```python
from build123d import *

# Parameters (mm, degrees)
F0_R         = 11.125
F1_DEPTH     = 10
F2_T1_DEPTH  = 17.5952575274
F2_T3_DEPTH  = 17.5952575274
F2_T6_ANGLE  = 359.64
F2_T8_ANGLE  = 359.64
F2_T10_ANGLE = 158.7108465942
F2_T12_ANGLE = 359.64
F2_T14_ANGLE = 359.64
F2_T16_ANGLE = 359.64
F2_T18_ANGLE = 359.64
F2_T20_ANGLE = 158.7108465942
F2_T22_ANGLE = 359.64
F2_T24_ANGLE = 359.64
F2_T26_ANGLE = 359.64
F2_T28_ANGLE = 158.7108465942
F2_T30_ANGLE = 359.64
F2_T32_ANGLE = 359.64
F2_T34_ANGLE = 359.64
F2_T36_ANGLE = 359.64
F2_T38_ANGLE = 359.64
F2_T40_ANGLE = 359.64
F2_T42_ANGLE = 158.7108465942
F2_T44_ANGLE = 359.64


# Not quite as in the source:
# - a fillet or chamfer that OpenCascade refuses, or shapes differently, is made with other operations: its cross-section is extruded or revolved along the edge and cut away or added


with BuildPart() as f1:
    # F0 (on Top) → F1 (new body)
    with BuildSketch(Plane.XY):
        with BuildLine():
            Line((-2.8125022072, -17.6151320338), (0, -17.6151320338))
            Line((0, -17.6151320338), (2.8125022072, -17.6151320338))
            Line((2.8125022072, -17.6151320338), (2.8125022072, -25.0164493918))
            Line((2.8125022072, -25.0164493918), (6.0690809041, -25.0164493918))
            Line((6.0690809041, -25.0164493918), (6.0690809041, -20.2796068043))
            ThreePointArc((6.0690809041, -20.2796068043), (11.9901318103, -14.3585558981), (17.9111827165, -20.2796068043))
            ThreePointArc((17.9111827165, -20.2796068043), (25.8046814323, -21.1516241303), (27.4031855301, -28.930603552))
            ThreePointArc((27.4031855301, -28.930603552), (43.3717109263, 0), (27.4031855301, 28.930603552))
            ThreePointArc((27.4031855301, 28.930603552), (25.8046814323, 21.1516241303), (17.9111827165, 20.2796068043))
            ThreePointArc((17.9111827165, 20.2796068043), (11.9901318103, 14.3585558981), (6.0690809041, 20.2796068043))
            Line((6.0690809041, 20.2796068043), (6.0690809041, 25.0164493918))
            Line((6.0690809041, 25.0164493918), (2.8125022072, 25.0164493918))
            Line((2.8125022072, 25.0164493918), (2.8125022072, 17.6151320338))
            Line((2.8125022072, 17.6151320338), (0, 17.6151320338))
            Line((0, 17.6151320338), (-2.8125022072, 17.6151320338))
            Line((-2.8125022072, 17.6151320338), (-2.8125022072, 25.0164493918))
            Line((-2.8125022072, 25.0164493918), (-6.0690809041, 25.0164493918))
            Line((-6.0690809041, 25.0164493918), (-6.0690809041, 20.2796068043))
            ThreePointArc((-6.0690809041, 20.2796068043), (-11.9901318103, 14.3585558981), (-17.9111827165, 20.2796068043))
            ThreePointArc((-17.9111827165, 20.2796068043), (-25.8046814323, 21.1516241303), (-27.4031855301, 28.930603552))
            ThreePointArc((-27.4031855301, 28.930603552), (-43.3717109263, 0), (-27.4031855301, -28.930603552))
            ThreePointArc((-27.4031855301, -28.930603552), (-25.8046814323, -21.1516241303), (-17.9111827165, -20.2796068043))
            ThreePointArc((-17.9111827165, -20.2796068043), (-11.9901318103, -14.3585558981), (-6.0690809041, -20.2796068043))
            Line((-6.0690809041, -20.2796068043), (-6.0690809041, -25.0164493918))
            Line((-6.0690809041, -25.0164493918), (-2.8125022072, -25.0164493918))
            Line((-2.8125022072, -25.0164493918), (-2.8125022072, -17.6151320338))
        make_face()
        Polygon((-30.9119913686, 5.5693711821), (-24.537748198, 5.4711418492), (-21.4356957103, -0.0982293328), (-24.7078863932, -5.5693711821), (-31.0821295639, -5.4711418492), (-34.1841820515, 0.0982293328), align=None, mode=Mode.SUBTRACT)
        Circle(F0_R, mode=Mode.SUBTRACT)
        Polygon((20.875, 0), (24.0625, 5.5209119491), (30.4375, 5.5209119491), (33.625, 0), (30.4375, -5.5209119491), (24.0625, -5.5209119491), align=None, mode=Mode.SUBTRACT)
    extrude(amount=F1_DEPTH)

    # F2: chamfer of 5 on 20 edges, made by hand

    # F2_s2 → F2_t1 (cut)
    with BuildSketch(Plane.XZ.offset(-37.8748643317)):
        Polygon((-6.0690809041, 5), (-1.0690809041, 0), (-6.0690809041, 0), align=None)
        Polygon((6.0690809041, 5), (1.0690809041, 0), (6.0690809041, 0), align=None)
        Polygon((1.0690809041, 10), (6.0690809041, 5), (6.0690809041, 10), align=None)
        Polygon((-1.0690809041, 10), (-6.0690809041, 5), (-6.0690809041, 10), align=None)
    extrude(amount=F2_T1_DEPTH, mode=Mode.SUBTRACT)

    # F2_s4 → F2_t3 (cut)
    with BuildSketch(Plane.XZ.offset(20.2796068043)):
        Polygon((-1.0690809041, 0), (-6.0690809041, 5), (-6.0690809041, 0), align=None)
        Polygon((6.0690809041, 5), (1.0690809041, 0), (6.0690809041, 0), align=None)
        Polygon((1.0690809041, 10), (6.0690809041, 5), (6.0690809041, 10), align=None)
        Polygon((-1.0690809041, 10), (-6.0690809041, 5), (-6.0690809041, 10), align=None)
    extrude(amount=F2_T3_DEPTH, mode=Mode.SUBTRACT)

    # F2_s5 → F2_t6 (revolve, cut)
    with BuildSketch(Plane(origin=(-24.5672156268, 22.5322183518, 0), x_dir=(0, 0, 1), z_dir=(-0.7369707586, 0.6759246267, 0))):
        Polygon((10, 16.6434047939), (5, 11.6434047939), (10, 11.6434047939), align=None)
    revolve(axis=Axis((-21.2587402157, 26.1394987159, 10), (0, 0, -1)), revolution_arc=F2_T6_ANGLE, mode=Mode.SUBTRACT)

    # F2_s7 → F2_t8 (revolve, cut)
    with BuildSketch(Plane.XZ.offset(-20.2796068043)):
        Polygon((-1.0690809041, 10), (-6.0690809041, 5), (-6.0690809041, 10), align=None)
    revolve(axis=Axis((-11.9901318103, 20.2796068043, 10), (0, 0, -1)), revolution_arc=F2_T8_ANGLE, mode=Mode.SUBTRACT)

    # F2_s9 → F2_t10 (revolve, cut)
    with BuildSketch(Plane(origin=(-8.8670439331, -1.6665634724, 0), x_dir=(0, 0, 1), z_dir=(0.9827919356, 0.1847160286, 0))):
        Polygon((10, -30.8871798498), (5, -35.8871798498), (10, -35.8871798498), align=None)
    revolve(axis=Axis((-9.1802750199, 0, 10), (0, 0, 1)), revolution_arc=F2_T10_ANGLE, mode=Mode.SUBTRACT)

    # F2_s11 → F2_t12 (revolve, cut)
    with BuildSketch(Plane(origin=(-24.6850209159, -22.3563277123, 0), x_dir=(0, 0, 1), z_dir=(0.7412031432, 0.6712807911, 0))):
        Polygon((10, 16.8527592984), (5, 11.8527592984), (10, 11.8527592984), align=None)
    revolve(axis=Axis((-21.2587402157, -26.1394987159, 10), (0, 0, -1)), revolution_arc=F2_T12_ANGLE, mode=Mode.SUBTRACT)

    # F2_s13 → F2_t14 (revolve, cut)
    with BuildSketch(Plane(origin=(-0.1278905192, -20.3541404453, 0), x_dir=(0, 0, 1), z_dir=(0.006283144, 0.9999802609, 0))):
        Polygon((5, -5.9414245401), (10, -0.9414245401), (10, -5.9414245401), align=None)
    revolve(axis=Axis((-11.9901318103, -20.2796068043, 10), (0, 0, -1)), revolution_arc=F2_T14_ANGLE, mode=Mode.SUBTRACT)

    # F2_s15 → F2_t16 (revolve, cut)
    with BuildSketch(Plane.XZ.offset(20.2796068043)):
        Polygon((1.0690809041, 10), (6.0690809041, 5), (6.0690809041, 10), align=None)
    revolve(axis=Axis((11.9901318103, -20.2796068043, 10), (0, 0, -1)), revolution_arc=F2_T16_ANGLE, mode=Mode.SUBTRACT)

    # F2_s17 → F2_t18 (revolve, cut)
    with BuildSketch(Plane(origin=(24.5672156268, -22.5322183518, 0), x_dir=(0, 0, 1), z_dir=(0.7369707586, -0.6759246267, 0))):
        Polygon((10, 16.6434047939), (5, 11.6434047939), (10, 11.6434047939), align=None)
    revolve(axis=Axis((21.2587402157, -26.1394987159, 10), (0, 0, -1)), revolution_arc=F2_T18_ANGLE, mode=Mode.SUBTRACT)

    # F2_s19 → F2_t20 (revolve, cut)
    with BuildSketch(Plane(origin=(8.8670439331, 1.6665634724, 0), x_dir=(0, 0, 1), z_dir=(-0.9827919356, -0.1847160286, 0))):
        Polygon((10, -30.8871798498), (5, -35.8871798498), (10, -35.8871798498), align=None)
    revolve(axis=Axis((9.1802750199, 0, 10), (0, 0, 1)), revolution_arc=F2_T20_ANGLE, mode=Mode.SUBTRACT)

    # F2_s21 → F2_t22 (revolve, cut)
    with BuildSketch(Plane(origin=(24.6850209159, 22.3563277123, 0), x_dir=(0, 0, 1), z_dir=(-0.7412031432, -0.6712807911, 0))):
        Polygon((10, 16.8527592984), (5, 11.8527592984), (10, 11.8527592984), align=None)
    revolve(axis=Axis((21.2587402157, 26.1394987159, 10), (0, 0, -1)), revolution_arc=F2_T22_ANGLE, mode=Mode.SUBTRACT)

    # F2_s23 → F2_t24 (revolve, cut)
    with BuildSketch(Plane(origin=(0.1278905192, 20.3541404453, 0), x_dir=(0, 0, 1), z_dir=(-0.006283144, -0.9999802609, 0))):
        Polygon((10, -0.9414245401), (5, -5.9414245401), (10, -5.9414245401), align=None)
    revolve(axis=Axis((11.9901318103, 20.2796068043, 10), (0, 0, -1)), revolution_arc=F2_T24_ANGLE, mode=Mode.SUBTRACT)

    # F2_s25 → F2_t26 (revolve, cut)
    with BuildSketch(Plane(origin=(24.6850209159, 22.3563277123, 0), x_dir=(0, 0, 1), z_dir=(-0.7412031432, -0.6712807911, 0))):
        Polygon((5, 11.8527592984), (0, 16.8527592984), (0, 11.8527592984), align=None)
    revolve(axis=Axis((21.2587402157, 26.1394987159, 0), (0, 0, -1)), revolution_arc=F2_T26_ANGLE, mode=Mode.SUBTRACT)

    # F2_s27 → F2_t28 (revolve, cut)
    with BuildSketch(Plane(origin=(8.8670439331, 1.6665634724, 0), x_dir=(0, 0, 1), z_dir=(-0.9827919356, -0.1847160286, 0))):
        Polygon((5, -35.8871798498), (0, -30.8871798498), (0, -35.8871798498), align=None)
    revolve(axis=Axis((9.1802750199, 0, 0), (0, 0, 1)), revolution_arc=F2_T28_ANGLE, mode=Mode.SUBTRACT)

    # F2_s29 → F2_t30 (revolve, cut)
    with BuildSketch(Plane(origin=(24.5672156268, -22.5322183518, 0), x_dir=(0, 0, 1), z_dir=(0.7369707586, -0.6759246267, 0))):
        Polygon((5, 11.6434047939), (0, 16.6434047939), (0, 11.6434047939), align=None)
    revolve(axis=Axis((21.2587402157, -26.1394987159, 0), (0, 0, -1)), revolution_arc=F2_T30_ANGLE, mode=Mode.SUBTRACT)

    # F2_s31 → F2_t32 (revolve, cut)
    with BuildSketch(Plane.XZ.offset(20.2796068043)):
        Polygon((6.0690809041, 5), (1.0690809041, 0), (6.0690809041, 0), align=None)
    revolve(axis=Axis((11.9901318103, -20.2796068043, 0), (0, 0, -1)), revolution_arc=F2_T32_ANGLE, mode=Mode.SUBTRACT)

    # F2_s33 → F2_t34 (revolve, cut)
    with BuildSketch(Plane(origin=(-0.1278905192, -20.3541404453, 0), x_dir=(0, 0, 1), z_dir=(0.006283144, 0.9999802609, 0))):
        Polygon((5, -5.9414245401), (0, -0.9414245401), (0, -5.9414245401), align=None)
    revolve(axis=Axis((-11.9901318103, -20.2796068043, 0), (0, 0, -1)), revolution_arc=F2_T34_ANGLE, mode=Mode.SUBTRACT)

    # F2_s35 → F2_t36 (revolve, cut)
    with BuildSketch(Plane(origin=(0.1278905192, 20.3541404453, 0), x_dir=(0, 0, 1), z_dir=(-0.006283144, -0.9999802609, 0))):
        Polygon((5, -5.9414245401), (0, -0.9414245401), (0, -5.9414245401), align=None)
    revolve(axis=Axis((11.9901318103, 20.2796068043, 0), (0, 0, -1)), revolution_arc=F2_T36_ANGLE, mode=Mode.SUBTRACT)

    # F2_s37 → F2_t38 (revolve, cut)
    with BuildSketch(Plane.XZ.offset(-20.2796068043)):
        Polygon((-6.0690809041, 5), (-1.0690809041, 0), (-6.0690809041, 0), align=None)
    revolve(axis=Axis((-11.9901318103, 20.2796068043, 0), (0, 0, -1)), revolution_arc=F2_T38_ANGLE, mode=Mode.SUBTRACT)

    # F2_s39 → F2_t40 (revolve, cut)
    with BuildSketch(Plane(origin=(-24.5672156268, 22.5322183518, 0), x_dir=(0, 0, 1), z_dir=(-0.7369707586, 0.6759246267, 0))):
        Polygon((5, 11.6434047939), (0, 16.6434047939), (0, 11.6434047939), align=None)
    revolve(axis=Axis((-21.2587402157, 26.1394987159, 0), (0, 0, -1)), revolution_arc=F2_T40_ANGLE, mode=Mode.SUBTRACT)

    # F2_s41 → F2_t42 (revolve, cut)
    with BuildSketch(Plane(origin=(-8.8670439331, -1.6665634724, 0), x_dir=(0, 0, 1), z_dir=(0.9827919356, 0.1847160286, 0))):
        Polygon((5, -35.8871798498), (0, -30.8871798498), (0, -35.8871798498), align=None)
    revolve(axis=Axis((-9.1802750199, 0, 0), (0, 0, 1)), revolution_arc=F2_T42_ANGLE, mode=Mode.SUBTRACT)

    # F2_s43 → F2_t44 (revolve, cut)
    with BuildSketch(Plane(origin=(-24.6850209159, -22.3563277123, 0), x_dir=(0, 0, 1), z_dir=(0.7412031432, 0.6712807911, 0))):
        Polygon((0, 16.8527592984), (5, 11.8527592984), (0, 11.8527592984), align=None)
    revolve(axis=Axis((-21.2587402157, -26.1394987159, 0), (0, 0, -1)), revolution_arc=F2_T44_ANGLE, mode=Mode.SUBTRACT)


solid = f1.part
```
Part model, mm, in its own coordinate system. A direction names the side the tool comes from. Coordinates: 2 decimals unless noted, no trailing zeros. Loops run counter-clockwise (first coordinate to the right, second up) from the corner with the lowest first, then second, coordinate; pieces in that order, holes last. Notation, with made-up numbers: (56, 22) - (75, 22) arc R26 ccw to (75, 49) - close; hole circle Ø7 at (-12, 85.25). An arc over 180 degrees is marked (long way). Write item = value, one per line. Start each with the question number.
Item 1: Cut at B-B, the plane y = -15.5. State how many separate pieces and enclosed holes the cut face has, and give its area (3 significant figures).
Item 2: Cut at A-A, the plane x = 0. Give the cut face in (y, z) (3 decimals), and give its area (3 significant figures).
Item 3: 3-axis set-ups, long thin cutter, end or side, ignore diameter. For faces 1 (the flat face through (2.813, -21, 5)), 2 (the flat face through (32.01, 2.8, 4.93)), 3 (the flat face through (4.46, -22.61, 3.39)), 4 (the flat face through (-2.813, 21, 5)): which of +Z, -Z, +X, -X, +Y, -Y reach the whole face in a straight line?
Item 4: Flat gauge pins, fed straight in: pin 1 Ø1.6 at (x, z) = (-4, 5) entering from +Y; pin 2 Ø5 at (x, z) = (34.5, 4.5) entering from -Y; pin 3 Ø10 at (x, y) = (2, -0.5) entering from +Z; pin 4 Ø1.5 at (y, z) = (-12, 7) entering from +X. Where does each tip first touch, or does it go through?
Item 5: Wall check: L1, parallel to Y at x = 0, z = 8 (3 decimals); L2, parallel to X at y = -22.5, z = 6.5; L3, parallel to X at y = -15, z = 4.75. Give the ranges that are in metal, low to high. Write a range as from..to.
The answers:
q1.separate_pieces = 3
q1.enclosed_holes = 0
q1.area = 447 mm2
q2.outline = (-17.615, 0) - (-11.125, 0) - (-11.125, 10) - (-17.615, 10) - close; (11.125, 0) - (17.615, 0) - (17.615, 10) - (11.125, 10) - close
q2.area = 130 mm2
q3.face_1 = +Z, -Z, -Y
q3.face_2 = +Z, -Z
q3.face_3 = -Z, -Y
q3.face_4 = +Z, -Z, +Y
q4.pin_1 = 25.02
q4.pin_2 = -25.42
q4.pin_3 = through
q4.pin_4 = 39.91
q5.L1 = -17.615..-11.125, 11.125..17.615
q5.L2 = -32.9..-28.66, -4.57..-2.81, 2.81..4.57, 28.66..32.9
q5.L3 = -39.63..-15.19, -8.8..8.8, 15.19..39.63
